```python
from build123d import *

# Parameters (mm, degrees)
F0_W      = 50.8
F0_H      = 50.8
F1_DEPTH  = 7.62
F2_T      = -1.27
F3_W      = 1.27
F3_H      = 43.18
F4_DEPTH  = 7.62
F5_W      = 1.27
F5_H      = 26.6756825149
F6_DEPTH  = 7.62
F7_W      = 1.27
F7_H      = 25.4
F8_DEPTH  = 7.62
F9_W      = 17.78
F9_H      = 1.27
F10_DEPTH = 7.62
F11_W     = 1.27
F11_H     = 25.4
F12_DEPTH = 7.62
F13_W     = 12.7
F13_H     = 1.27
F14_DEPTH = 7.62
F15_W     = 15.9816620052
F15_H     = 1.27
F16_DEPTH = 7.62
F17_W     = 25.4
F17_H     = 1.27
F18_DEPTH = 7.62
F19_R     = 1.27
F20_DEPTH = 203.2


# Not quite as in the source:
# - a feature names something its author has since deleted; it is built from what else it names


with BuildPart() as f1:
    # F0 (on Top) → F1 (new body)
    with BuildSketch(Plane.XY):
        with Locations((25.4, 25.4)):
            Rectangle(F0_W, F0_H)
    extrude(amount=-F1_DEPTH)

    # F2
    f2_openings = [f1.faces().sort_by_distance(p)[0] for p in [
        (25.4, 25.4, 0),
    ]]
    offset(amount=F2_T, openings=f2_openings)

    # F3 (on face) → F4 (join)
    with BuildSketch(Plane.XY.offset(-6.35)):
        with Locations((6.985, 22.86)):
            Rectangle(F3_W, F3_H)
    extrude(amount=F4_DEPTH)

    # F5 (on Top) → F6 (join)
    with BuildSketch(Plane.XY):
        with Locations((15.1333379948, 36.3023299724)):
            Rectangle(F5_W, F5_H)
    extrude(amount=-F6_DEPTH)

    # F7 (on face) → F8 (join)
    with BuildSketch(Plane.XY.offset(-6.35)):
        with Locations((21.4833379948, 13.97)):
            Rectangle(F7_W, F7_H)
    extrude(amount=F8_DEPTH)

    # F9 (on face) → F10 (join)
    with BuildSketch(Plane.XY.offset(-6.35)):
        with Locations((24.6583379948, 32.385)):
            Rectangle(F9_W, F9_H)
    extrude(amount=F10_DEPTH)

    # F11 (on face) → F12 (join)
    with BuildSketch(Plane.XY.offset(-6.35)):
        with Locations((27.8333379948, 19.05)):
            Rectangle(F11_W, F11_H)
    extrude(amount=F12_DEPTH)

    # F13 (on face) → F14 (join)
    with BuildSketch(Plane.XY.offset(-6.35)):
        with Locations((34.8183379948, 26.035)):
            Rectangle(F13_W, F13_H)
    extrude(amount=F14_DEPTH)

    # F15 (on face) → F16 (join)
    with BuildSketch(Plane.XY.offset(-6.35)):
        with Locations((36.4591689974, 7.9343094056)):
            Rectangle(F15_W, F15_H)
    extrude(amount=F16_DEPTH)

    # F17 (on face) → F18 (join)
    with BuildSketch(Plane.XY.offset(-6.35)):
        with Locations((36.83, 43.815)):
            Rectangle(F17_W, F17_H)
    extrude(amount=F18_DEPTH)

    # F19 (on face) → F20 (cut)
    with BuildSketch(Plane.XY.offset(-6.35)):
        with Locations((3.6000448745, 4.547465127)):
            Circle(F19_R)
        with Locations((3.8395691663, 10.7227088884)):
            Circle(F19_R)
        with Locations((19.5783379948, 36.2029448152)):
            Circle(F19_R)
        with Locations((31.4771048725, 16.6409648955)):
            Circle(F19_R)
    extrude(amount=-F20_DEPTH, mode=Mode.SUBTRACT)


solid = f1.part
```
Part model, mm, in its own coordinate system. A direction names the side the tool comes from. Coordinates: 2 decimals unless noted, no trailing zeros. Order: outer loops, then holes, each group sorted by start corner. A loop starts at its lowest first (then second) coordinate and runs counter-clockwise, first axis right, second up. Notation, with made-up numbers: (30.5, 69) -> (41.5, 69) arc R17 ccw to (41.5, 89) -> close; hole circle Ø3 at (51, 2.5). An arc over 180 degrees is marked (long way). Put each result on its own line as item: value. Start each with the question number.
(1) Band-saw the part on B-B (y = 29). Give the cut face in (x, z), then the cut area to 3 significant figures.
(2) Pin check, flat tips, straight feed: pin 1 Ø1 at (x, y) = (41, 14.5) entering from +Z; pin 2 Ø1.5 at (x, y) = (3.6, 4.55) entering from +Z (3 decimals). Stop position of each tip, or through.
(3) Mould opens along Y. For faces 1 (the face through (37, 43.18, -3)), 2 (the face through (15.768, 32, 1)), 3 (the face through (25, 0, -4)), 4 (the face through (32, 49.53, -3)) say: pulls with the +Y half, pulls with the -Y half, needs draft (parallel to the pull), parting line crosses it, or undercut.
(4) Which spindle directions (+Z, -Z, +X, -X, +Y, -Y) get a long thin tool onto all of the face, cutting with end or side? Do faces 5 (the face through (23, 1, 0)), 6 (the face through (25, 26, -7.62)). Say none if no direction does.
(5) Band-saw the part on C-C (x = 46). Give the cut face in (y, z), then the cut area to 3 significant figures.
(6) Probe line 1 along Y through (x, z) = (29, -5.75); line 2 along X through (y, z) = (23.5, -4.5); line 3 along X through (y, z) = (8.5, -0.25). List the from-to ranges inside material, lowest first. Write a range as [from, to].
(7) Band-saw the part on A-A (x = 11). Give the cut face in (y, z), then the cut area to 3 significant figures.
Determined:
1. outline: (0, -7.62) -> (50.8, -7.62) -> (50.8, 0) -> (49.53, 0) -> (49.53, -6.35) -> (28.47, -6.35) -> (28.47, 1.27) -> (27.2, 1.27) -> (27.2, -6.35) -> (15.77, -6.35) -> (15.77, 0) -> (14.5, 0) -> (14.5, -6.35) -> (7.62, -6.35) -> (7.62, 1.27) -> (6.35, 1.27) -> (6.35, -6.35) -> (1.27, -6.35) -> (1.27, 0) -> (0, 0) -> close
1. area: 108 mm²
2. pin 1: stops at z = -6.35
2. pin 2: passes through
3. face 1: undercut
3. face 2: needs draft
3. face 3: pulls with the -Y half
3. face 4: undercut
4. face 5: +Z
4. face 6: -Z, +X, -X, +Y, -Y
5. outline: (0, -7.62) -> (50.8, -7.62) -> (50.8, 0) -> (49.53, 0) -> (49.53, -6.35) -> (44.45, -6.35) -> (44.45, 1.27) -> (43.18, 1.27) -> (43.18, -6.35) -> (1.27, -6.35) -> (1.27, 0) -> (0, 0) -> close
5. area: 90.3 mm²
6. line 1: y = [0, 1.27], [7.3, 8.57], [25.4, 26.67], [31.75, 33.02], [43.18, 44.45], [49.53, 50.8]
6. line 2: x = [0, 1.27], [6.35, 7.62], [14.5, 15.77], [20.85, 22.12], [27.2, 28.47], [49.53, 50.8]
6. line 3: x = [0, 1.27], [6.35, 7.62], [20.85, 22.12], [27.2, 44.45], [49.53, 50.8]
7. outline: (0, -7.62) -> (50.8, -7.62) -> (50.8, 0) -> (49.53, 0) -> (49.53, -6.35) -> (1.27, -6.35) -> (1.27, 0) -> (0, 0) -> close
7. area: 80.6 mm²
